Here's how the part is built. I have some questions about the finished solid (model axes, mm). Round coordinates to 2 decimals unless told otherwise and drop trailing zeros. Loops run counter-clockwise (first coordinate to the right, second up) from the corner with the lowest first, then second, coordinate; pieces in that order, holes last. Notation, with made-up numbers: (-36, 17) -> (-30, 17) arc R23 cw to (-30, 47) -> close; hole circle Ø3 at (42.5, 37.25). An arc over 180 degrees is marked (long way). Use one line per item in the form item = value. Start each with the question number.
Item 1: If we section it at B-B (y = 3.5): Write out the boundary of the cut face in (x, z).
Item 2: If I drill on L1, parallel to Z at x = -1.5, y = -4.75; L2, parallel to X at y = -2.25, z = 0.45, over which ranges is the centre line in solid material (lowest first)? Write a range as [from, to].
Item 3: If we section it at A-A (x = -0.75): Write out the boundary of the cut face in (y, z), then the cut area to 3 significant figures.
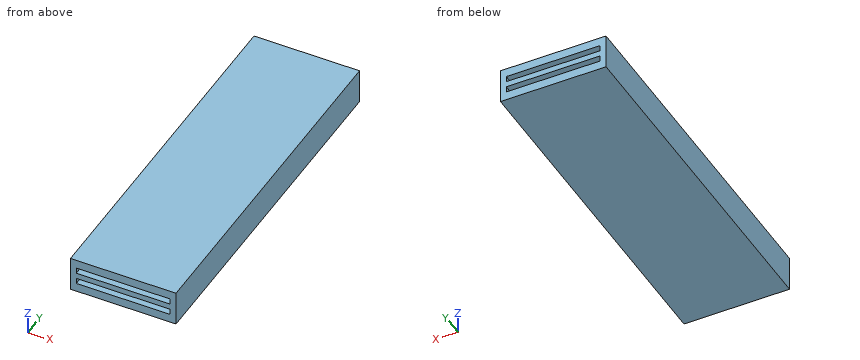
```python
from build123d import *

# Parameters (mm, degrees)
SKETCH1_W           = 9
SKETCH1_H           = 3
BOSS_EXTRUDE1_DEPTH = 15
CUT_EXTRUDE1_START  = -31
SKETCH2_W           = 8
SKETCH2_H           = 0.5
CUT_EXTRUDE1_DEPTH  = 32


with BuildPart() as part:
    # Sketch1 → Boss-Extrude1 (new body, symmetric)
    with BuildSketch(Plane(origin=(0, 0, 0), x_dir=(1, 0, 0), z_dir=(0, 1, 0))):
        Rectangle(SKETCH1_W, SKETCH1_H)
    extrude(amount=BOSS_EXTRUDE1_DEPTH, both=True)

    # Sketch2 → Cut-Extrude1 (cut)
    with BuildSketch(Plane(origin=(0, 15, 0), x_dir=(1, 0, 0), z_dir=(0, 1, 0)).offset(CUT_EXTRUDE1_START)):
        with Locations((0, 0.5)):
            Rectangle(SKETCH2_W, SKETCH2_H)
    cut_extrude1 = extrude(amount=CUT_EXTRUDE1_DEPTH, mode=Mode.SUBTRACT)

    # Mirror1: Cut-Extrude1 across plane
    add(cut_extrude1.mirror(Plane.XY), mode=Mode.SUBTRACT)


solid = part.part
```
Values found:
q1.outline = (-4.5, -1.5) -> (4.5, -1.5) -> (4.5, 1.5) -> (-4.5, 1.5) -> close; hole (-4, -0.75) -> (4, -0.75) -> (4, -0.25) -> (-4, -0.25) -> close; hole (-4, 0.25) -> (4, 0.25) -> (4, 0.75) -> (-4, 0.75) -> close
q2.L1 = [-1.5, -0.75], [-0.25, 0.25], [0.75, 1.5]
q2.L2 = [-4.5, -4], [4, 4.5]
q3.outline = (-15, -1.5) -> (15, -1.5) -> (15, -0.75) -> (-15, -0.75) -> close; (-15, -0.25) -> (15, -0.25) -> (15, 0.25) -> (-15, 0.25) -> close; (-15, 0.75) -> (15, 0.75) -> (15, 1.5) -> (-15, 1.5) -> close
q3.area = 60.0 mm2
